Model file for the job. Use its own axes, mm. A direction names the side the tool comes from. Coordinates: 2 decimals unless noted, no trailing zeros. Loops run counter-clockwise (first coordinate to the right, second up) from the corner with the lowest first, then second, coordinate; pieces in that order, holes last. Notation, with made-up numbers: (-8.5, 11.5) -> (4.5, 11.5) arc R20 ccw to (4.5, 50.5) -> close; hole circle Ø4 at (-38.75, 13.25). An arc over 180 degrees is marked (long way). Use one line per item in the form item = value.
```python
from build123d import *

# Parameters (mm, degrees)
SKETCH7_R           = 7
BOSS_EXTRUDE2_DEPTH = 30
CHAMFER2_SIZE       = 1


with BuildPart() as part:
    # Sketch6 → Revolve2 (revolve)
    with BuildSketch(Plane.XZ):
        Polygon((30, 75), (0, 75), (0, 0), (53, 0), (53, 5), (110, 5), (110, 30), (30, 30), align=None)
    revolve(axis=Axis((0, 0, 75), (0, 0, -1)))

    # Sketch7 → Boss-Extrude2 (add)
    with BuildSketch(Plane(origin=(0, 0, 5), x_dir=(-1, 0, 0), z_dir=(0, 0, -1))):
        with Locations((-57.629202667, -57.629202667)):
            Circle(SKETCH7_R)
        with Locations((-81.5, 0)):
            Circle(SKETCH7_R)
        with Locations((-57.629202667, 57.629202667)):
            Circle(SKETCH7_R)
        with Locations((0, 81.5)):
            Circle(SKETCH7_R)
        with Locations((57.629202667, 57.629202667)):
            Circle(SKETCH7_R)
        with Locations((81.5, 0)):
            Circle(SKETCH7_R)
        with Locations((0, -81.5)):
            Circle(SKETCH7_R)
        with Locations((57.629202667, -57.629202667)):
            Circle(SKETCH7_R)
    extrude(amount=BOSS_EXTRUDE2_DEPTH)

    # Chamfer2
    chamfer2_edges = [part.edges().sort_by_distance(p)[0] for p in [
        (64.629202667, -57.629202667, -25),
        (88.5, 0, -25),
        (64.629202667, 57.629202667, -25),
        (7, 81.5, -25),
        (-50.629202667, 57.629202667, -25),
        (7, -81.5, -25),
        (-74.5, 0, -25),
        (-50.629202667, -57.629202667, -25),
    ]]
    chamfer(chamfer2_edges, length=CHAMFER2_SIZE)


solid = part.part
```
Q1. Band-saw the part on D-D, the plane z = 50.5. Write the cut outline in (x, y), and give its area (3 significant figures).
Result:
outline = circle Ø60 at (0, 0)
area = 2,830 mm2
Q2. Pin check, flat tips, straight feed: pin 1 Ø2 at (x, y) = (63, -43) entering from +Z; pin 2 Ø10 at (x, y) = (22, 22) entering from -Z; pin 3 Ø4 at (x, y) = (80, -79.5) entering from +Z; pin 4 Ø5 at (x, z) = (43.5, 29.5) entering from +Y. Stop position of each tip, or through.
Result:
pin_1 = 30
pin_2 = 0
pin_3 = through
pin_4 = 102.07
Q3. Which spindle directions (+Z, -Z, +X, -X, +Y, -Y) get a long thin tool onto all of the face, cutting with end or side? Do faces 1 (the face through (23, 23, 30)), 2 (the face through (-23.846, 107.384, 17.675)), 3 (the face through (1, -1, 0)). Say none if no direction does.
Result:
face_1 = +Z
face_2 = +Z, -Z
face_3 = -Z
Q4. Band-saw the part on B-B, the plane z = -15.5. Write the cut outline in (x, y).
Result:
outline = circle Ø14 at (-81.5, 0); circle Ø14 at (-57.63, -57.63); circle Ø14 at (-57.63, 57.63); circle Ø14 at (0, -81.5); circle Ø14 at (0, 81.5); circle Ø14 at (57.63, -57.63); circle Ø14 at (57.63, 57.63); circle Ø14 at (81.5, 0)
Q5. Band-saw the part on A-A, the plane y = 0. Write the cut outline in (x, z), and give its area (3 significant figures).
Result:
outline = (-110, 5) -> (-88.5, 5) -> (-88.5, -24) -> (-87.5, -25) -> (-75.5, -25) -> (-74.5, -24) -> (-74.5, 5) -> (-53, 5) -> (-53, 0) -> (53, 0) -> (53, 5) -> (74.5, 5) -> (74.5, -24) -> (75.5, -25) -> (87.5, -25) -> (88.5, -24) -> (88.5, 5) -> (110, 5) -> (110, 30) -> (30, 30) -> (30, 75) -> (-30, 75) -> (-30, 30) -> (-110, 30) -> close
area = 9,570 mm2
Q6. Band-saw the part on C-C, the plane x = 20. Write the cut outline in (y, z), and give its area (3 significant figures).
Result:
outline = (-108.17, 5) -> (-49.08, 5) -> (-49.08, 0) -> (49.08, 0) -> (49.08, 5) -> (108.17, 5) -> (108.17, 30) -> (22.36, 30) -> (22.36, 75) -> (-22.36, 75) -> (-22.36, 30) -> (-108.17, 30) -> close
area = 7,910 mm2
Q7. Mould opens along Y. For faces 4 (the face through (-74.507, 0.308, -9.297)), 5 (the face through (-58, -58, -25)), 6 (the face through (54.4, -63.84, -9.3)) say: released by +Y, released by -Y, zero draft, split by the parting line, or undercut.
Result:
face_4 = split by the parting line
face_5 = zero draft
face_6 = undercut
Q8. Wall check: line 1 along X through (y, z) = (-0.5, 27); line 2 along Z through (x, y) = (32.5, -80.5); line 3 along X through (y, z) = (1, 34). Give the ranges that are in metal, low to high.
Result:
line_1 = -110 to 110
line_2 = 5 to 30
line_3 = -29.98 to 29.98
